Geometry check sheet. Reference: drawing and pictorial views, mm from the part's lowest x, y, z. A direction names the side the tool comes from. Give positions to 0.01 mm unless a question says otherwise; leave off trailing zeros. Loops run counter-clockwise (first coordinate to the right, second up) from the corner with the lowest first, then second, coordinate; pieces in that order, holes last. Notation, with made-up numbers: (-9, 58.25) - (26, 58.25) arc R9 ccw to (26, 71.25) - close; hole circle Ø7 at (26.25, -6.75). An arc over 180 degrees is marked (long way). Use CSV: the item, a comma, the result in double quotes.
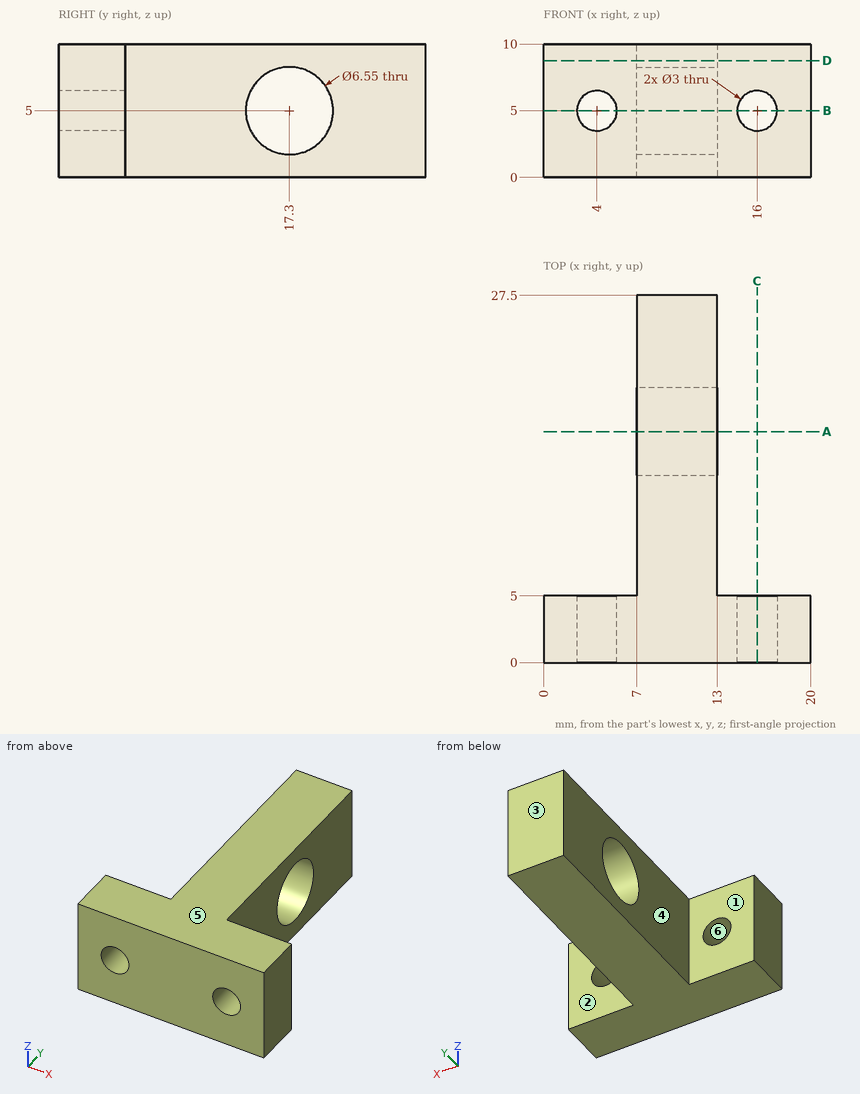
1. Scan lines: line 1 along Z through (x, y) = (4, 1.9); line 2 along X through (y, z) = (2.5, 3.75); line 3 along X through (y, z) = (1, 4.25). Record each from-to range of solid material in increasing order.
Completed:
line 1,"z = 0 to 3.5, 6.5 to 10"
line 2,"x = 0 to 3.17, 4.83 to 15.17, 16.83 to 20"
line 3,"x = 0 to 2.7, 5.3 to 14.7, 17.3 to 20"
2. Sectioned sample at B-B, the plane z = 5. Record the boundary of the cut face in (x, y) (3 decimals), and give its area (3 significant figures).
Completed:
outline,"(0, 0) - (2.5, 0) - (2.5, 5) - (0, 5) - close; (5.5, 0) - (14.5, 0) - (14.5, 5) - (13, 5) - (13, 14.025) - (7, 14.025) - (7, 5) - (5.5, 5) - close; (7, 20.575) - (13, 20.575) - (13, 27.5) - (7, 27.5) - close; (17.5, 0) - (20, 0) - (20, 5) - (17.5, 5) - close"
area,"166 mm²"
3. Set-up check for the marked faces 1, 2 and 3: record each of +Z, -Z, +X, -X, +Y, -Y from which the full face is reachable in a straight line by a thin tool's end or side.
Completed:
face 1,"+Z, -Z, -X, +Y"
face 2,"+Z, -Z, +X, +Y"
face 3,"+Z, -Z, +X, -X, +Y"
4. Go/stop test with flat-tipped pins: pin 1 Ø1.5 at (y, z) = (13.5, 3.5) entering from -X; pin 2 Ø5 at (x, z) = (16, 5) entering from +Y; pin 3 Ø5 at (y, z) = (14, 9) entering from +X. Record where each tip stops, or that it passes through.
Completed:
pin 1,"stops at x = 7"
pin 2,"stops at y = 5"
pin 3,"stops at x = 13"
5. Sectioned sample at D-D, the plane z = 8.75. Record the boundary of the cut face in (x, y).
Completed:
outline,"(0, 0) - (20, 0) - (20, 5) - (13, 5) - (13, 27.5) - (7, 27.5) - (7, 5) - (0, 5) - close"
6. Release check for a two-part mould opening along Z. For the marked faces 4, 5 and 6 record: released by +Z, released by -Z, zero draft, split by the parting line, or undercut.
Completed:
face 4,"zero draft"
face 5,"released by +Z"
face 6,"undercut"
7. Sectioned sample at A-A, the plane y = 17.3. Record the boundary of the cut face in (x, z) (3 decimals).
Completed:
outline,"(7, 0) - (13, 0) - (13, 1.725) - (7, 1.725) - close; (7, 8.275) - (13, 8.275) - (13, 10) - (7, 10) - close"
8. Sectioned sample at C-C, the plane x = 16. Record the boundary of the cut face in (y, z).
Completed:
outline,"(0, 0) - (5, 0) - (5, 3.5) - (0, 3.5) - close; (0, 6.5) - (5, 6.5) - (5, 10) - (0, 10) - close"
